from build123d import *

# Parameters (mm, degrees)
SCHIZZO2_R                   = 0.75
SCHIZZO2_R_2                 = 1.5
ESTRUSIONE_ESTRUSIONE1_DEPTH = 1.9
SCHIZZO3_R                   = 3.5
SCHIZZO3_R_2                 = 2.307795375
ESTRUSIONE_ESTRUSIONE2_DEPTH = 2.5


with BuildPart() as part:
    # Schizzo2 → Estrusione-Estrusione1 (new body)
    with BuildSketch(Plane.XY):
        with BuildLine():
            Line((0.477386935, 3.769894125), (20.063316583, 1.289700622))
            ThreePointArc((20.063316583, 1.289700622), (21.2, 0), (20.063316583, -1.289700622))
            Line((20.063316583, -1.289700622), (0.477386935, -3.769894125))
            ThreePointArc((0.477386935, -3.769894125), (-3.8, 0), (0.477386935, 3.769894125))
        make_face()
        with Locations((19.9, 0)):
            Circle(SCHIZZO2_R, mode=Mode.SUBTRACT)
        with Locations((6.7, 0)):
            Circle(SCHIZZO2_R, mode=Mode.SUBTRACT)
        with Locations((10, 0)):
            Circle(SCHIZZO2_R, mode=Mode.SUBTRACT)
        with Locations((13.3, 0)):
            Circle(SCHIZZO2_R, mode=Mode.SUBTRACT)
        with Locations((16.6, 0)):
            Circle(SCHIZZO2_R, mode=Mode.SUBTRACT)
        Circle(SCHIZZO2_R_2, mode=Mode.SUBTRACT)
    extrude(amount=ESTRUSIONE_ESTRUSIONE1_DEPTH)

    # Schizzo3 → Estrusione-Estrusione2 (add)
    with BuildSketch(Plane.XY):
        Circle(SCHIZZO3_R)
        Circle(SCHIZZO3_R_2, mode=Mode.SUBTRACT)
    extrude(amount=-ESTRUSIONE_ESTRUSIONE2_DEPTH)


solid = part.part
Source: CAD feature listing. Evaluate the final solid. Frame: model axes, mm. A direction names the side the tool comes from. Coordinates: 2 decimals unless noted, no trailing zeros. Order: outer loops, then holes, each group sorted by start corner. A loop starts at its lowest first (then second) coordinate and runs counter-clockwise, first axis right, second up.
Item 1: Pull-direction query (Y, two-part tool) for faces 1 (the face through (6, -1, 1.9)), 2 (the face through (9.25, 0.03, 0.94)), 3 (the face through (-3.8, -0.1, 0.9)); classes: pulls with the +Y half, pulls with the -Y half, needs draft (parallel to the pull), parting line crosses it, or undercut.
Output values:
face 1: needs draft
face 2: undercut
face 3: parting line crosses it
Item 2: Material intervals for line 1 (Z direction, x = 11, y = 1); line 2 (Y direction, x = 16.75, z = 0.8); line 3 (Y direction, x = 13.3, z = 1.2), sorted ascending.
Output values:
line 1: z = 0 to 1.9
line 2: y = -1.71 to -0.73, 0.73 to 1.71
line 3: y = -2.15 to -0.75, 0.75 to 2.15
Item 3: Cut plane B-B (z = 1). Return loops of the section in (x, y).
Output values:
outline: (0.48, -3.77) - (20.06, -1.29) arc R1.3 ccw to (20.06, 1.29) - (0.48, 3.77) arc R3.8 ccw (long way) to start; hole circle Ø3 at (0, 0); hole circle Ø1.5 at (6.7, 0); hole circle Ø1.5 at (10, 0); hole circle Ø1.5 at (13.3, 0); hole circle Ø1.5 at (16.6, 0); hole circle Ø1.5 at (19.9, 0)
Item 4: Cut plane A-A (x = 0). Return loops of the section in (y, z).
Output values:
outline: (-3.8, 0) - (-3.5, 0) - (-3.5, -2.5) - (-2.31, -2.5) - (-2.31, 0) - (-1.5, 0) - (-1.5, 1.9) - (-3.8, 1.9) - close; (1.5, 0) - (2.31, 0) - (2.31, -2.5) - (3.5, -2.5) - (3.5, 0) - (3.8, 0) - (3.8, 1.9) - (1.5, 1.9) - close
Item 5: Set-up query: faces 4 (the face through (-2, 0, 0)), 5 (the face through (20.615, 0.225, 0.937)). Return all of +Z, -Z, +X, -X, +Y, -Y with unobstructed straight access to the full face (end or side cutting, diameter ignored); none if empty.
Output values:
face 4: -Z
face 5: +Z, -Z
Item 6: Cut plane D-D (y = -3.25). Return loops of the section in (x, z), plus the area to 3 significant figures.
Output values:
outline: (-1.97, 0) - (-1.3, 0) - (-1.3, -2.5) - (1.3, -2.5) - (1.3, 0) - (4.58, 0) - (4.58, 1.9) - (-1.97, 1.9) - close
area: 18.9 mm2
Item 7: Cut plane C-C (z = -0.9). Return loops of the section in (x, y).
Output values:
outline: circle Ø7 at (0, 0); hole circle Ø4.62 at (0, 0)
Item 8: First-contact query: P1, Ø4, axis at x = 12, y = 0.5, coming from the -Z side; P2, Ø1.5, axis at y = -1, z = 0.5, coming from the +X side. Flat tips, straight axial feed; report the tip coordinate or a pass-through.
Output values:
P1: stops at z = 0
P2: stops at x = 21.18
